Source: CAD feature listing. Evaluate the final solid. Frame: model axes, mm. Give positions to 0.01 mm unless a question says otherwise; leave off trailing zeros. Loops run counter-clockwise (first coordinate to the right, second up) from the corner with the lowest first, then second, coordinate; pieces in that order, holes last. Notation, with made-up numbers: (-36.75, 59) -> (-20.75, 59) arc R25 cw to (-20.75, 91) -> close; hole circle Ø9 at (11.5, 1). An arc over 180 degrees is marked (long way). Put each result on its own line as item: value.
```python
from build123d import *

# Parameters (mm, degrees)
SKETCH1_W            = 85
SKETCH1_H            = 140
BOSS_EXTRUDE1_DEPTH  = 3.75
SKETCH2_R            = 2.5
CUT_EXTRUDE1_DEPTH   = 83.234421017
LPATTERN1_COUNT      = 3
LPATTERN1_PITCH      = 32.5
LPATTERN1_COUNT_DIR2 = 4
LPATTERN1_PITCH_DIR2 = 40


with BuildPart() as part:
    # Sketch1 → Boss-Extrude1 (new, symmetric)
    with BuildSketch(Plane.XY):
        Rectangle(SKETCH1_W, SKETCH1_H)
    extrude(amount=BOSS_EXTRUDE1_DEPTH, both=True)

    # Sketch2 → Cut-Extrude1 (cut, symmetric)
    with BuildSketch(Plane.XY.offset(3.75)):
        with Locations((-32.5, 60)):
            Circle(SKETCH2_R)
    cut_extrude1 = extrude(amount=CUT_EXTRUDE1_DEPTH, both=True, mode=Mode.SUBTRACT)

    # LPattern1: Cut-Extrude1 3 × 4, 4 skipped
    with Locations(*[(i * LPATTERN1_PITCH, -j * LPATTERN1_PITCH_DIR2, 0) for i in range(LPATTERN1_COUNT) for j in range(LPATTERN1_COUNT_DIR2) if (i, j) not in ((0, 0), (1, 1), (1, 2), (2, 1), (2, 2))]):
        add(cut_extrude1, mode=Mode.SUBTRACT)


solid = part.part
```
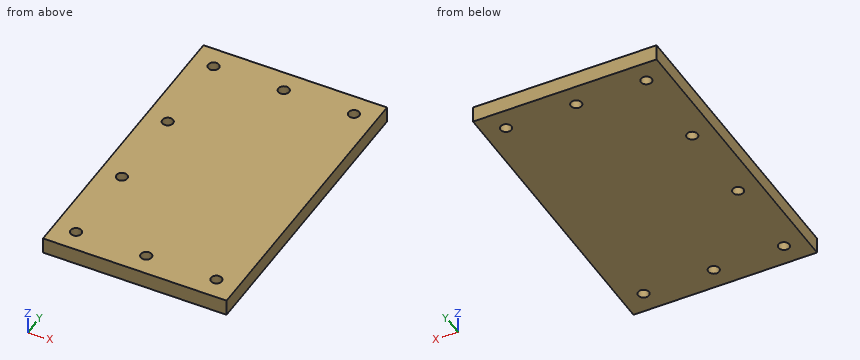
(1) Line query: probe 1 along Y at (x, z) = (32.5, -2); probe 2 along Y at (x, z) = (-32.5, -0.5); probe 3 along Y at (x, z) = (-0.5, -0.25). Output: solid intervals per line, ascending. Write a range as from..to.
Calculated:
probe 1: y = -70..-62.5, -57.5..57.5, 62.5..70
probe 2: y = -70..-62.5, -57.5..-22.5, -17.5..17.5, 22.5..57.5, 62.5..70
probe 3: y = -70..-62.45, -57.55..57.55, 62.45..70
(2) Section A-A on x = -32.5. Return loops of the section in (y, z), then the cut area to 3 significant figures.
Calculated:
outline: (-70, -3.75) -> (-62.5, -3.75) -> (-62.5, 3.75) -> (-70, 3.75) -> close; (-57.5, -3.75) -> (-22.5, -3.75) -> (-22.5, 3.75) -> (-57.5, 3.75) -> close; (-17.5, -3.75) -> (17.5, -3.75) -> (17.5, 3.75) -> (-17.5, 3.75) -> close; (22.5, -3.75) -> (57.5, -3.75) -> (57.5, 3.75) -> (22.5, 3.75) -> close; (62.5, -3.75) -> (70, -3.75) -> (70, 3.75) -> (62.5, 3.75) -> close
area: 900 mm²
(3) Section B-B on y = 60. Return loops of the section in (x, z).
Calculated:
outline: (-42.5, -3.75) -> (-35, -3.75) -> (-35, 3.75) -> (-42.5, 3.75) -> close; (-30, -3.75) -> (-2.5, -3.75) -> (-2.5, 3.75) -> (-30, 3.75) -> close; (2.5, -3.75) -> (30, -3.75) -> (30, 3.75) -> (2.5, 3.75) -> close; (35, -3.75) -> (42.5, -3.75) -> (42.5, 3.75) -> (35, 3.75) -> close
(4) First-contact query: P1, Ø3, axis at x = -32.5, y = 20, coming from the +Z side. Flat tip, straight axial feed; report the tip coordinate or a pass-through.
Calculated:
P1: passes through
(5) Section D-D on y = 20. Return loops of the section in (x, z).
Calculated:
outline: (-42.5, -3.75) -> (-35, -3.75) -> (-35, 3.75) -> (-42.5, 3.75) -> close; (-30, -3.75) -> (42.5, -3.75) -> (42.5, 3.75) -> (-30, 3.75) -> close
(6) Section C-C on x = 32.5. Return loops of the section in (y, z).
Calculated:
outline: (-70, -3.75) -> (-62.5, -3.75) -> (-62.5, 3.75) -> (-70, 3.75) -> close; (-57.5, -3.75) -> (57.5, -3.75) -> (57.5, 3.75) -> (-57.5, 3.75) -> close; (62.5, -3.75) -> (70, -3.75) -> (70, 3.75) -> (62.5, 3.75) -> close
